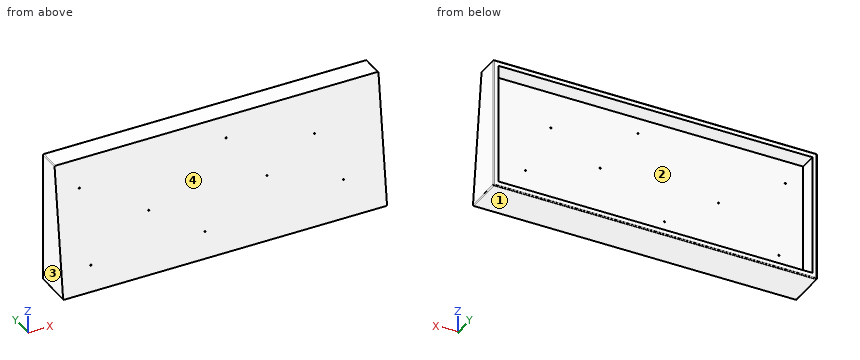
from build123d import *

# Parameters (mm, degrees)
SKETCH1_W             = 320
SKETCH1_H             = 130
BOSS_EXTRUDE3_DEPTH   = 22
SKETCH3_W             = 310
SKETCH3_H             = 120
CUT_EXTRUDE1_DEPTH    = 17
DRAFT1_ANGLE          = 7
FILLET2_R             = 1
F_0_80_TAPPED_HOLE1_D = 1.19126


with BuildPart() as part:
    # Sketch1 → Boss-Extrude3 (new body)
    with BuildSketch(Plane(origin=(0, 0, 0), x_dir=(1, 0, 0), z_dir=(0, 1, 0))):
        with Locations((160, 65)):
            Rectangle(SKETCH1_W, SKETCH1_H)
    extrude(amount=BOSS_EXTRUDE3_DEPTH)

    # Sketch3 → Cut-Extrude1 (cut)
    with BuildSketch(Plane(origin=(0, 22, 0), x_dir=(1, 0, 0), z_dir=(0, 1, 0))):
        with Locations((160, 65)):
            Rectangle(SKETCH3_W, SKETCH3_H)
    extrude(amount=-CUT_EXTRUDE1_DEPTH, mode=Mode.SUBTRACT)

    # Draft1
    draft1_faces = [part.faces().sort_by_distance(p)[0] for p in [
        (160, 0, -65),
    ]]
    draft(draft1_faces, Plane(origin=(0, 22, 0), x_dir=(1, 0, 0), z_dir=(0, 0, 1)), DRAFT1_ANGLE)

    # Fillet2
    fillet2_edges = [part.edges().sort_by_distance(p)[0] for p in [
        (320, 22, -65),
        (160, 22, -130),
        (0, 22, -65),
        (0, 3.019003541, -130),
        (320, 3.019003541, -130),
        (320, 11, 0),
        (0, 11, 0),
        (160, 22, 0),
    ]]
    fillet(fillet2_edges, radius=FILLET2_R)

    # #0-80 Tapped Hole1 (through all)
    with Locations(Plane(origin=(28.97111002, 5, -104.431910758), x_dir=(0, 0, 1), z_dir=(0, 1, 0))):
        with Locations((0, 0), (0.301233355, 112.962508169), (36.148002614, 59.644204314), (36.449235969, 176.522746099), (63.259004574, 225.322549628), (11.446867494, 250.324918103), (76.513272199, -6.325900457), (83.742872722, 139.169810064)):
            Hole(F_0_80_TAPPED_HOLE1_D / 2)


solid = part.part
The model under review builds one solid part; all positions refer to its coordinate system, in mm. Face numbers are marked on the shaded views. Round coordinates to 2 decimals unless told otherwise and drop trailing zeros. Order: outer loops, then holes, each group sorted by start corner. A loop starts at its lowest first (then second) coordinate and runs counter-clockwise, first axis right, second up. Notation, with made-up numbers: (89.25, 72.25) -> (138.25, 72.25) arc R27 cw to (138.25, 108.25) -> close; hole circle Ø3 at (-5.75, -37.75). An arc over 180 degrees is marked (long way). Return JSON: item names as keys, results as strings.
1. Take a section at C-C (z = -113.5). Write out the cut boundary in (x, y), then the cut area to 3 significant figures.
Answer block:
{"outline": "(0, -13.94) -> (320, -13.94) -> (320, 21) arc R1 ccw to (319, 22) -> (315, 22) -> (315, 5) -> (5, 5) -> (5, 22) -> (1, 22) arc R1 ccw to (0, 21) -> close", "area": "6,230 mm²"}
2. Take a section at B-B (x = 36). Write out the cut boundary in (y, z), then the cut area to 3 significant figures.
Answer block:
{"outline": "(-15.96, -130) -> (21, -130) arc R1 ccw to (22, -129) -> (22, -125) -> (5, -125) -> (5, -5) -> (22, -5) -> (22, -1) arc R1 ccw to (21, 0) -> (0, 0) -> close", "area": "1,860 mm²"}
3. For L1, parallel to X at y = 19, z = -64; L2, parallel to Z at x = 145, y = 6; L3, parallel to Y at x = 257, z = -68.5, list the stretches that pass through material, from the lowest coordinate up. Write a range as [from, to].
Answer block:
{"L1": "x = [0, 5], [315, 320]", "L2": "z = [-130, -125], [-5, 0]", "L3": "y = [-8.41, 5]"}
4. Insertion check: P1, Ø1.5, axis at x = 168.14, z = -20.69, coming from the +Y side; P2, Ø1.9, axis at x = 141.93, z = -104.13, coming from the -Y side; P3, Ø1.5, axis at x = 128, z = -19, coming from the -Y side (3 decimals). Each pin has a flat end and moves straight along its axis. Give the tip position at first contact, or say it passes through.
Answer block:
{"P1": "stops at y = 5", "P2": "stops at y = -12.9", "P3": "stops at y = -2.425"}
5. The part is to be moulded in two halves that separate along Z. For the marked faces 1, 2, 3 and 4, say which applies: +Z half, -Z half, draft (parallel to the pull), parting line (faces both ways), or undercut.
Answer block:
{"face 1": "-Z half", "face 2": "undercut", "face 3": "draft", "face 4": "+Z half"}
6. Take a section at A-A (y = 17). Write out the cut boundary in (x, z), then the cut area to 3 significant figures.
Answer block:
{"outline": "(0, -129) arc R1 ccw to (1, -130) -> (319, -130) arc R1 ccw to (320, -129) -> (320, -1) arc R1 ccw to (319, 0) -> (1, 0) arc R1 ccw to (0, -1) -> close; hole (5, -125) -> (315, -125) -> (315, -5) -> (5, -5) -> close", "area": "4,400 mm²"}
